Input: part model. Units: mm. Frame: model coordinates. A direction names the side the tool comes from. Coordinates: 2 decimals unless noted, no trailing zeros. Order: outer loops, then holes, each group sorted by start corner. A loop starts at its lowest first (then second) coordinate and runs counter-clockwise, first axis right, second up. Notation, with made-up numbers: (62.5, 31.25) -> (92.5, 31.25) arc R23 ccw to (92.5, 54.25) -> close; hole circle Ø7 at (-16.5, 37.5). An arc over 180 degrees is marked (long way). Answer as CSV lines item,"result".
from build123d import *

# Parameters (mm, degrees)
F0_W      = 140
F0_H      = 60
F1_DEPTH  = 35
F3_DEPTH  = 140.001
F4_W      = 30
F4_H      = 30
F5_DEPTH  = 60
F6_R      = 20
F7_DEPTH  = 72.1
F9_DEPTH  = 10
F11_DEPTH = 25
F12_R     = 5
F13_DEPTH = 25


# Not quite as in the source:
# - a pattern or mirror of a feature is missing from the dataset's text; its kind, count and spacing are read off the source's solid


with BuildPart() as f1:
    # F0 (on Front) → F1 (new body, symmetric)
    with BuildSketch(Plane.XZ):
        Rectangle(F0_W, F0_H)
    extrude(amount=F1_DEPTH, both=True)

    # F2 (on face) → F3 (cut, through all)
    with BuildSketch(Plane.YZ.offset(70)):
        with BuildLine():
            Line((-20, -30), (20, -30))
            ThreePointArc((20, -30), (0, -10), (-20, -30))
        make_face()
        with BuildLine():
            ThreePointArc((-20, -30), (0, -50), (20, -30))
            Line((20, -30), (-20, -30))
        make_face()
    extrude(amount=-F3_DEPTH, mode=Mode.SUBTRACT)

    # F4 (on face) → F5 (cut)
    with BuildSketch(Plane.XZ.offset(35)):
        with Locations((55, 15)):
            Rectangle(F4_W, F4_H)
    f5 = extrude(amount=-F5_DEPTH, mode=Mode.SUBTRACT)

    # F5_copies: F5 across plane
    add(f5.mirror(Plane(origin=(0, 0, 0), x_dir=(0, 0, -1), z_dir=(-1, 0, 0))), mode=Mode.SUBTRACT)

    # F6 (on face) → F7 (cut)
    with BuildSketch(Plane.XZ.offset(35)):
        with Locations((0, 30)):
            Circle(F6_R)
    extrude(amount=-F7_DEPTH, mode=Mode.SUBTRACT)

    # F8 (on face) → F9 (join)
    with BuildSketch(Plane.XZ.offset(35)):
        with BuildLine():
            Line((0, 30), (-30, 30))
            ThreePointArc((-30, 30), (0, 0), (30, 30))
            Line((30, 30), (0, 30))
        make_face()
    extrude(amount=F9_DEPTH)

    # F10 (on face) → F11 (cut)
    with BuildSketch(Plane(origin=(0, -35, 0), x_dir=(-1, 0, 0), z_dir=(0, 1, 0))):
        with BuildLine():
            ThreePointArc((-20, 30), (0, 10), (20, 30))
            Line((20, 30), (-20, 30))
        make_face()
    extrude(amount=-F11_DEPTH, mode=Mode.SUBTRACT)

    # F12 (on face) → F13 (cut)
    with BuildSketch(Plane.XZ.offset(-25)):
        with Locations((55, 15)):
            Circle(F12_R)
    f13 = extrude(amount=-F13_DEPTH, mode=Mode.SUBTRACT)

    # F13_copies: F13 across plane
    add(f13.mirror(Plane(origin=(0, 0, 0), x_dir=(0, 0, -1), z_dir=(-1, 0, 0))), mode=Mode.SUBTRACT)

    # F15: F1 across plane


with BuildPart() as f1_1:
    add(f1.part)
    add(f1.part.mirror(Plane.XY.offset(30)))


solid = f1_1.part
1. Cut plane C-C (y = -0.5). Return the cut outline in (x, z).
Findings:
outline,"(-70, -10.01) -> (70, -10.01) -> (70, 0) -> (40, 0) -> (40, 60) -> (70, 60) -> (70, 70.01) -> (-70, 70.01) -> (-70, 60) -> (-40, 60) -> (-40, 0) -> (-70, 0) -> close; hole circle Ø40 at (0, 30)"
2. Cut plane D-D (z = -21.5). Return the cut outline in (x, y), plus the area to 3 significant figures.
Findings:
outline,"(-70, -35) -> (70, -35) -> (70, -18.1) -> (-70, -18.1) -> close; (-70, 18.1) -> (70, 18.1) -> (70, 35) -> (-70, 35) -> close"
area,"4,730 mm2"
3. Cut plane B-B (z = 45). Return the cut outline in (x, y).
Findings:
outline,"(-70, 25) -> (-60, 25) -> (-60, 35) -> (-70, 35) -> close; (-50, 25) -> (-40, 25) -> (-40, -35) -> (-25.98, -35) -> (-25.98, -45) -> (-13.23, -45) -> (-13.23, 35) -> (-50, 35) -> close; (13.23, -45) -> (25.98, -45) -> (25.98, -35) -> (40, -35) -> (40, 25) -> (50, 25) -> (50, 35) -> (13.23, 35) -> close; (60, 25) -> (70, 25) -> (70, 35) -> (60, 35) -> close"
4. Ray query, line 1 along Z through (x, y) = (-55, 30.25); line 2 along Z through (x, y) = (56.5, 29.5); line 3 along X through (y, z) = (31.5, 45). Return the intervals inside material, ascending.
Findings:
line 1,"z = -30 to 10, 20 to 40, 50 to 90"
line 2,"z = -30 to 10.23, 19.77 to 40.23, 49.77 to 90"
line 3,"x = -70 to -60, -50 to -13.23, 13.23 to 50, 60 to 70"
5. Cut plane A-A (x = 0). Return the cut outline in (y, z), plus the area to 3 significant figures.
Findings:
outline,"(-45, 0) -> (-35, 0) -> (-35, -30) -> (-20, -30) arc R20 cw to (20, -30) -> (35, -30) -> (35, 10) -> (-45, 10) -> close; (-45, 50) -> (35, 50) -> (35, 90) -> (20, 90) arc R20 cw to (-20, 90) -> (-35, 90) -> (-35, 60) -> (-45, 60) -> close"
area,"4,540 mm2"
6. Reachability of faces 1 (the face through (-1, -28, -30)), 2 (the face through (55, 25, 30)), 3 (the face through (-55, 25, 30)) from +Z, -Z, +X, -X, +Y, -Y: full face, straight path, thin tool, end or side. Return the list, or none.
Findings:
face 1,"-Z, +X, -X, +Y, -Y"
face 2,"+X, -Y"
face 3,"-X, -Y"
7. Contact query for flat-ended pins moving along their axis: pin 1 (3 mm diameter, centred on y = 14.5, z = 2, fed in from -X); pin 2 (9 mm diameter, centred on x = 50.5, z = 41.5, fed in from -Y); pin 3 (9 mm diameter, centred on x = 55, z = 15, fed in from +Y); pin 4 (15 mm diameter, centred on x = 61.5, y = -0.5, fed in from -Z). Output: stop coordinate, or through.
Findings:
pin 1,"stops at x = -40"
pin 2,"stops at y = 25"
pin 3,"passes through"
pin 4,"stops at z = -11.67"
8. Mould query, pull axis X, two halves, no side actions, for faces 4 (the face through (70, 31, 31)), 5 (the face through (-2.6, -5.56, 10.17)), 6 (the face through (-17, -35, 2)). Classes: released by +X, released by -X, zero draft, split by the parting line, or undercut.
Findings:
face 4,"released by +X"
face 5,"undercut"
face 6,"zero draft"
